Geometry: see drawing. Coordinates: mm, zero at the bounding-box minimum. A direction names the side the tool comes from. Give positions to 0.01 mm unless a question says otherwise; leave off trailing zeros. Order: outer loops, then holes, each group sorted by start corner. A loop starts at its lowest first (then second) coordinate and runs counter-clockwise, first axis right, second up. Notation, with made-up numbers: (-31, -21) - (-18, -21) arc R24 ccw to (-18, 4) - close; hole circle Ø1 at (54, 72.5). An arc over 180 degrees is marked (long way). Put each result on its own line as item: value. Start each with the question number.
1. Section C-C on z = 7.75. Return the cut outline in (x, y), plus the area to 3 significant figures.
2. Ray query, line 1 along Z through (x, y) = (4, 1.25); line 2 along Z through (x, y) = (6.5, 1.5); line 3 along X through (y, z) = (4.75, 5.5). Return the intervals inside material, ascending. Write a range as from..to.
3. First-contact query: P1, Ø3, axis at x = 6, y = 3.5, coming from the -Z side; P2, Ø1.5, axis at x = 3, z = 9, coming from the +Y side. Flat tips, straight axial feed; report the tip coordinate or a pass-through.
4. Section D-D on y = 1.75. Return the cut outline in (x, z), plus the area to 3 significant figures.
5. Set-up query: the marked faces 1, 2 and 3. Return all of +Z, -Z, +X, -X, +Y, -Y with unobstructed straight access to the full face (end or side cutting, diameter ignored); none if empty.
6. Section B-B on x = 4. Return the cut outline in (y, z).
7. Section A-A on y = 4. Return the cut outline in (x, z).
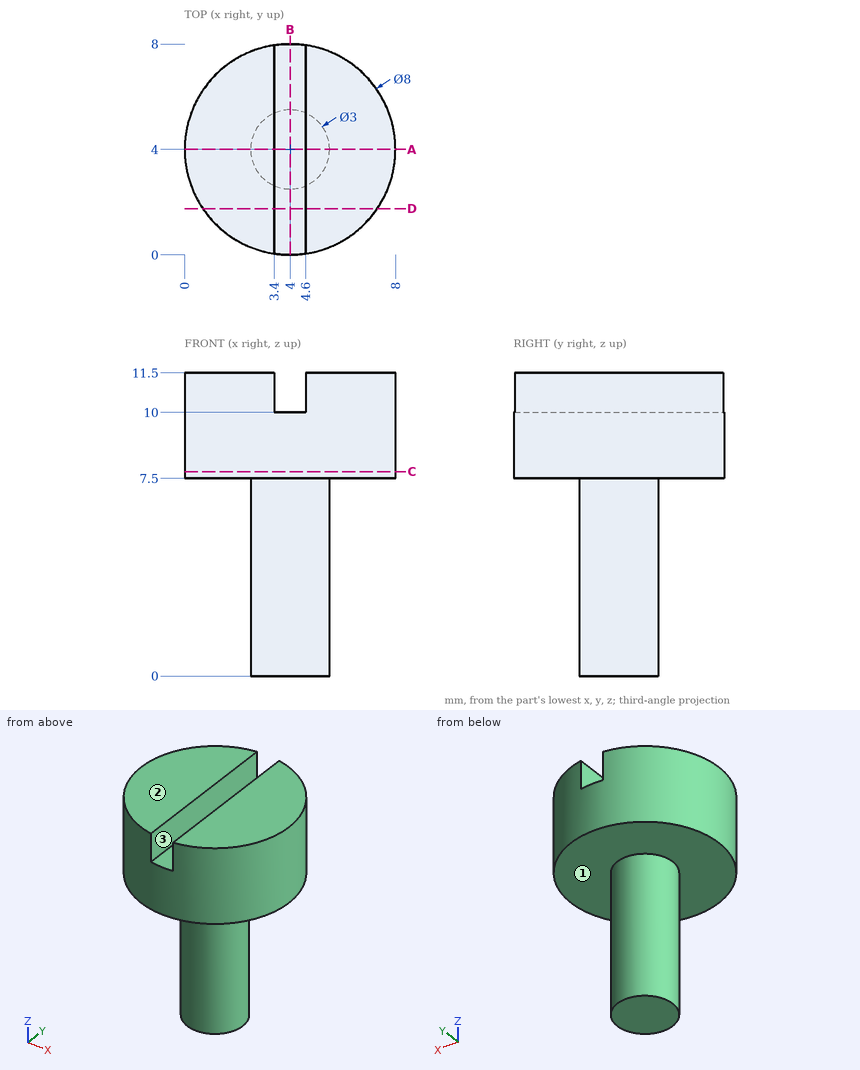
Resolved:
1. outline: circle Ø8 at (4, 4)
1. area: 50.3 mm^2
2. line 1: 7.5..10
2. line 2: 7.5..11.5
2. line 3: 2.7..5.3
3. P1: z = 0
3. P2: y = 7.99
4. outline: (0.69, 7.5) - (7.31, 7.5) - (7.31, 11.5) - (4.6, 11.5) - (4.6, 10) - (3.4, 10) - (3.4, 11.5) - (0.69, 11.5) - close
4. area: 24.7 mm^2
5. face 1: -Z
5. face 2: +Z, +X, -X, +Y, -Y
5. face 3: +Z, +Y, -Y
6. outline: (0, 7.5) - (2.5, 7.5) - (2.5, 0) - (5.5, 0) - (5.5, 7.5) - (8, 7.5) - (8, 10) - (0, 10) - close
7. outline: (0, 7.5) - (2.5, 7.5) - (2.5, 0) - (5.5, 0) - (5.5, 7.5) - (8, 7.5) - (8, 11.5) - (4.6, 11.5) - (4.6, 10) - (3.4, 10) - (3.4, 11.5) - (0, 11.5) - close
